Read the model definition and answer for the solid it produces. Units are mm, in the model's axes. A direction names the side the tool comes from. Round coordinates to 2 decimals unless told otherwise and drop trailing zeros. Order: outer loops, then holes, each group sorted by start corner. A loop starts at its lowest first (then second) coordinate and runs counter-clockwise, first axis right, second up. Notation, with made-up numbers: (-19, -8.75) -> (-7, -8.75) arc R14 ccw to (-7, 18.25) -> close; hole circle Ø10 at (70, 60.25). An arc over 180 degrees is marked (long way). One line per item, written item: value. Start each with the question number.
1. For faces 4 (the face through (-6, -17, 0)), 5 (the face through (6.5, -2, 0)), determine the directions among +Z, -Z, +X, -X, +Y, -Y from which every point of the face is accessible in a straight line to the end or side of a thin tool.
2. Consider line 1 (Z direction, x = 0, y = -15.75); line 2 (Y direction, x = 2.5, z = -6); line 3 (X direction, y = -18, z = -2.25). Determine where each line is inside the solid, lowest interval first.
3. Flat-ended cylindrical pins translate along their axes: pin 1 Ø3 at (x, z) = (-1, 6) entering from +Y; pin 2 Ø4 at (x, z) = (0, 0) entering from -Y; pin 3 Ø4 at (x, z) = (3, 4) entering from +Y; pin 4 Ø4 at (x, y) = (2.5, 2.5) entering from -Z. Find the tip coordinate at first contact, or state that the pin passes through.
4. The mould has two halves that part along X. Classify faces 1 (the face through (-0.45, -15.86, -3.425)), 2 (the face through (-3.78, 18.03, 2.9)), 3 (the face through (0, 31.4, 0)): released by +X, released by -X, zero draft, split by the parting line, or undercut.
5. Section A-A (y = -19) is taken. Give the vertices of the cut face in (x, z).
from build123d import *

# Parameters (mm, degrees)
SKETCH1_R                    = 4.7625
BOSS_EXTRUDE1_DEPTH          = 31.4
SKETCH3_R                    = 12.7
BOSS_EXTRUDE2_DEPTH          = 3
SKETCH4_R                    = 6
BOSS_EXTRUDE3_DEPTH          = 26
FILLET1_R                    = 6
F_5_16_24_TAPPED_HOLE1_D     = 6.9088
F_5_16_24_TAPPED_HOLE1_DEPTH = 20
F_5_16_24_TAPPED_HOLE1_TIP   = 2.075612922
SKETCH2_OUTSIDE_W            = 40.942
SKETCH2_OUTSIDE_H            = 40.942
CUT_EXTRUDE1_DEPTH           = 32.4
CUT_EXTRUDE1_DEPTH_BACK      = 27
CHAMFER1_SIZE                = 1


with BuildPart() as part:
    # Sketch1 → Boss-Extrude1 (new body)
    with BuildSketch(Plane(origin=(0, 0, 0), x_dir=(1, 0, 0), z_dir=(0, 1, 0))):
        Circle(SKETCH1_R)
    extrude(amount=BOSS_EXTRUDE1_DEPTH)

    # Sketch3 → Boss-Extrude2 (add)
    with BuildSketch(Plane(origin=(0, 0, 0), x_dir=(1, 0, 0), z_dir=(0, 1, 0))):
        Circle(SKETCH3_R)
    extrude(amount=-BOSS_EXTRUDE2_DEPTH)

    # Sketch4 → Boss-Extrude3 (add)
    with BuildSketch(Plane(origin=(0, 0, 0), x_dir=(1, 0, 0), z_dir=(0, 1, 0))):
        Circle(SKETCH4_R)
    extrude(amount=-BOSS_EXTRUDE3_DEPTH)

    # Fillet1
    fillet1_edges = [part.edges().sort_by_distance(p)[0] for p in [
        (-6, -3, 0),
        (-4.7625, 0, 0),
    ]]
    fillet(fillet1_edges, radius=FILLET1_R)

    # 5/16-24 Tapped Hole1
    with Locations(Plane(origin=(0, -26, 0), x_dir=(-1, 0, 0), z_dir=(0, -1, 0))):
        with Locations((0, 0)):
            Hole(F_5_16_24_TAPPED_HOLE1_D / 2, depth=F_5_16_24_TAPPED_HOLE1_DEPTH)
            with Locations((0, 0, -(F_5_16_24_TAPPED_HOLE1_DEPTH + F_5_16_24_TAPPED_HOLE1_TIP / 2))):  # 118° drill point
                Cone(0, F_5_16_24_TAPPED_HOLE1_D / 2, F_5_16_24_TAPPED_HOLE1_TIP, mode=Mode.SUBTRACT)

    # Sketch2 outside → Cut-Extrude1 (cut, two sides)
    with BuildSketch(Plane(origin=(0, 0, 0), x_dir=(1, 0, 0), z_dir=(0, 1, 0))) as cut_extrude1_sk:
        Rectangle(SKETCH2_OUTSIDE_W, SKETCH2_OUTSIDE_H)
        Polygon((6.5, -3.75277675), (6.5, 3.75277675), (0, 7.505553499), (-6.5, 3.75277675), (-6.5, -3.75277675), (0, -7.505553499), align=None, mode=Mode.SUBTRACT)
    extrude(amount=CUT_EXTRUDE1_DEPTH, mode=Mode.SUBTRACT)
    extrude(cut_extrude1_sk.sketch, amount=-CUT_EXTRUDE1_DEPTH_BACK, mode=Mode.SUBTRACT)

    # Chamfer1
    chamfer1_edges = [part.edges().sort_by_distance(p)[0] for p in [
        (-4.7625, 31.4, 0),
    ]]
    chamfer(chamfer1_edges, length=CHAMFER1_SIZE)


solid = part.part
Answer:
1. face 4: -Y
1. face 5: +Z, -Z, +X, +Y, -Y
2. line 1: -6 to -3.45, 3.45 to 6
2. line 2: -6.6 to 1.78
2. line 3: -5.56 to -2.62, 2.62 to 5.56
3. pin 1: y = 30.58
3. pin 2: y = -5.13
3. pin 3: y = 31.4
3. pin 4: z = -6.98
4. face 1: undercut
4. face 2: split by the parting line
4. face 3: zero draft
5. outline: circle Ø12 at (0, 0); hole circle Ø6.91 at (0, 0)
